```python
from build123d import *

# Parameters (mm, degrees)
SKETCH1_W           = 8.39079
SKETCH1_H           = 17.612704871
SKETCH1_W_2         = 9.17363
BOSS_EXTRUDE1_DEPTH = 25
SKETCH2_R           = 2.9110285
CUT_EXTRUDE1_DEPTH  = 409.009554619
CUT_EXTRUDE2_DEPTH  = 409.009554619
SKETCH4_W           = 582.34
SKETCH4_H           = 123.66999206
CUT_EXTRUDE3_DEPTH  = 7
FILLET1_R           = 5
SKETCH5_W           = 582.34
SKETCH5_H           = 3.612357777
CUT_EXTRUDE4_DEPTH  = 307.667781892


with BuildPart() as part:
    # Sketch1 → Boss-Extrude1 (new body)
    with BuildSketch(Plane(origin=(0, 0, 0), x_dir=(1, 0, 0), z_dir=(0, 1, 0))):
        Polygon((291.17, 76.945), (-291.17, 76.945), (-291.17, -76.945), (-104.943162, -76.945), (-96.552372, -76.945), (-79.86659, -76.945), (-70.69296, -76.945), (70.69296, -76.945), (79.86659, -76.945), (96.552372, -76.945), (104.943162, -76.945), (291.17, -76.945), align=None)
        with Locations((100.747767, -85.751352436)):
            Rectangle(SKETCH1_W, SKETCH1_H)
        with Locations((75.279775, -85.751352436)):
            Rectangle(SKETCH1_W_2, SKETCH1_H)
        with Locations((-75.279775, -85.751352436)):
            Rectangle(SKETCH1_W_2, SKETCH1_H)
        with Locations((-100.747767, -85.751352436)):
            Rectangle(SKETCH1_W, SKETCH1_H)
    extrude(amount=BOSS_EXTRUDE1_DEPTH)

    # Sketch2 → Cut-Extrude1 (cut, through all)
    with BuildSketch(Plane(origin=(104.943162, 0, 0), x_dir=(0, 0, -1), z_dir=(1, 0, 0))):
        with Locations((-87.882438934, 8.748719463)):
            Circle(SKETCH2_R)
    extrude(amount=-CUT_EXTRUDE1_DEPTH, mode=Mode.SUBTRACT)

    # Sketch3 → Cut-Extrude2 (cut, through all)
    with BuildSketch(Plane(origin=(104.943162, 0, 0), x_dir=(0, 0, -1), z_dir=(1, 0, 0))):
        with BuildLine():
            Line((-76.945, 0), (-87.882438934, 2.073453526))
            ThreePointArc((-87.882438934, 2.073453526), (-92.59600701, 4.012761881), (-94.557704871, 8.717055919))
            Line((-94.557704871, 8.717055919), (-94.557704871, 0))
            Line((-94.557704871, 0), (-76.945, 0))
        make_face()
        Polygon((-94.557704871, 17.434111839), (-76.945, 25), (-94.557704871, 25), align=None)
    extrude(amount=-CUT_EXTRUDE2_DEPTH, mode=Mode.SUBTRACT)

    # Sketch4 → Cut-Extrude3 (cut)
    with BuildSketch(Plane(origin=(0, 25, 0), x_dir=(1, 0, 0), z_dir=(0, 1, 0))):
        with Locations((0, 15.117928008)):
            Rectangle(SKETCH4_W, SKETCH4_H)
    extrude(amount=-CUT_EXTRUDE3_DEPTH, mode=Mode.SUBTRACT)

    # Fillet1
    fillet1_edges = [part.edges().sort_by_distance(p)[0] for p in [
        (0, 25, 46.717068022),
    ]]
    fillet(fillet1_edges, radius=FILLET1_R)

    # Sketch5 → Cut-Extrude4 (cut, through all)
    with BuildSketch(Plane(origin=(0, 18, 0), x_dir=(1, 0, 0), z_dir=(0, 1, 0))):
        with Locations((0, 75.138821112)):
            Rectangle(SKETCH5_W, SKETCH5_H)
    extrude(amount=-CUT_EXTRUDE4_DEPTH, mode=Mode.SUBTRACT)


solid = part.part
```
Check sheet for the modelled part. Datum: model origin and axes. Units: mm. A direction names the side the tool comes from. Give positions to 0.01 mm unless a question says otherwise; leave off trailing zeros. Loops run counter-clockwise (first coordinate to the right, second up) from the corner with the lowest first, then second, coordinate; pieces in that order, holes last. Notation, with made-up numbers: M 65.5,52 L 117.5,52 A20 ccw 117.5,60 Z; hole C -24,60 d2. An arc over 180 degrees is marked long. Answer in a Markdown table with one row per item.
1) Tool access check on faces 1 (the face through (-75.216, 1.022, 82.337)), 2 (the face through (-88, 12, 76.945)), 3 (the face through (-4, 18, -14)), 4 (the face through (-4, 0, 1)), 5 (the face through (197, 12, 76.945)). Record the directions out of +Z, -Z, +X, -X, +Y, -Y that give a thin tool (end or side, any length) a straight path to the whole face; none if there is none.
Solutions:
| item | result |
|---|---|
| face 1 | +Z, +X, -X, -Y |
| face 2 | +Z, +Y, -Y |
| face 3 | -Z, +X, -X, +Y |
| face 4 | +Z, -Z, +X, -X, -Y |
| face 5 | +Z, +X, +Y, -Y |
2) Cross-section at B-B (z = -22). Enter the section's corners in (x, y).
Solutions:
| item | result |
|---|---|
| outline | M -291.17,0 L 291.17,0 L 291.17,18 L -291.17,18 Z |
3) Depth check by flat-ended pin: pin 1 (1 mm diameter, centred on x = -106, y = 20, fed in from -Z); pin 2 (6 mm diameter, centred on x = -227, z = -13.5, fed in from -Y); pin 3 (7.5 mm diameter, centred on x = 191.5, y = 12.5, fed in from +Z) (3 decimals); pin 4 (5.5 mm diameter, centred on y = 8.5, z = 87.5, fed in from +X). Enter the tip coordinate at first touch or a pass-through.
Solutions:
| item | result |
|---|---|
| pin 1 | stops at z = 46.72 |
| pin 2 | stops at y = 0 |
| pin 3 | stops at z = 76.945 |
| pin 4 | stops at x = 104.94 |
4) Mould release check, pull along X, two halves, no side actions. Record for faces 6 (the face through (-4, 25, 64)), 7 (the face through (-291.17, 10, 1)), 8 (the face through (-70.693, 12, 84)): released by +X, released by -X, zero draft, split by the parting line, or undercut.
Solutions:
| item | result |
|---|---|
| face 6 | zero draft |
| face 7 | released by -X |
| face 8 | undercut |
5) Cross-section at A-A (x = -3). Enter the section's corners in (y, z) (3 decimals).
Solutions:
| item | result |
|---|---|
| outline | M 0,-73.333 L 18,-73.333 L 18,46.717 L 20,46.717 A5 ccw 25,51.717 L 25,76.945 L 0,76.945 Z |
6) Thickness scan on line 1 (Z direction, x = 8, y = 9) (3 decimals); line 2 (Y direction, x = -152, z = 4.5); line 3 (Z direction, x = 40, y = 19) (3 decimals). Record the ranges inside material, lowest first.
Solutions:
| item | result |
|---|---|
| line 1 | z = -73.333 to 76.945 |
| line 2 | y = 0 to 18 |
| line 3 | z = 46.717 to 76.945 |
